The model under review builds one solid part; all positions refer to its coordinate system, in mm. Coordinates: 2 decimals unless noted, no trailing zeros. Put each result on its own line as item: value.
from build123d import *

# Parameters (mm, degrees)
SKETCH_1_R           = 2.1
SKETCH_1_R_2         = 3.15
EXTRUDE_1_DEPTH      = 5
SKETCH_2_OUTSIDE_W   = 463.828
SKETCH_2_OUTSIDE_H   = 463.828
SKETCH_2_OUTSIDE_W_2 = 280
SKETCH_2_OUTSIDE_H_2 = 360
CUT_EXTRUDE_2_DEPTH  = 10
SKETCH_3_R           = 2.1
CUT_EXTRUDE_3_DEPTH  = 229.089894559
CUT_EXTRUDE_5_DEPTH  = 10
FILLET_1_R           = 10


with BuildPart() as part:
    # 草图1 → 凸台-拉伸1 (new body)
    with BuildSketch(Plane(origin=(0, 0, 0), x_dir=(1, 0, 0), z_dir=(0, 1, 0))):
        Polygon((-180, -180), (180, -180), (180, -160), (141, -160), (141, -100), (180, -100), (180, -30), (141, -30), (141, 30), (180, 30), (180, 100), (141, 100), (141, 160), (180, 160), (180, 180), (-180, 180), (-180, 160), (-141, 160), (-141, 100), (-180, 100), (-180, 30), (-141, 30), (-141, -30), (-180, -30), (-180, -100), (-141, -100), (-141, -160), (-180, -160), align=None)
        with Locations(Location((-103, 145, 0), (0, 0, 270))):
            Circle(SKETCH_1_R, mode=Mode.SUBTRACT)
        with Locations(Location((-103, 115, 0), (0, 0, 90))):
            Circle(SKETCH_1_R, mode=Mode.SUBTRACT)
        with Locations(Location((-127, 145, 0), (0, 0, 90))):
            Circle(SKETCH_1_R, mode=Mode.SUBTRACT)
        with Locations(Location((-127, 115, 0), (0, 0, 270))):
            Circle(SKETCH_1_R, mode=Mode.SUBTRACT)
        with Locations(Location((103, 145, 0), (0, 0, 270))):
            Circle(SKETCH_1_R, mode=Mode.SUBTRACT)
        with Locations(Location((103, 115, 0), (0, 0, 90))):
            Circle(SKETCH_1_R, mode=Mode.SUBTRACT)
        with Locations(Location((127, 145, 0), (0, 0, 90))):
            Circle(SKETCH_1_R, mode=Mode.SUBTRACT)
        with Locations(Location((127, 115, 0), (0, 0, 270))):
            Circle(SKETCH_1_R, mode=Mode.SUBTRACT)
        with Locations(Location((127, -115, 0), (0, 0, 270))):
            Circle(SKETCH_1_R, mode=Mode.SUBTRACT)
        with Locations(Location((127, -145, 0), (0, 0, 90))):
            Circle(SKETCH_1_R, mode=Mode.SUBTRACT)
        with Locations(Location((103, -145, 0), (0, 0, 270))):
            Circle(SKETCH_1_R, mode=Mode.SUBTRACT)
        with Locations(Location((103, -115, 0), (0, 0, 90))):
            Circle(SKETCH_1_R, mode=Mode.SUBTRACT)
        with Locations(Location((-127, -115, 0), (0, 0, 270))):
            Circle(SKETCH_1_R, mode=Mode.SUBTRACT)
        with Locations(Location((-103, -115, 0), (0, 0, 90))):
            Circle(SKETCH_1_R, mode=Mode.SUBTRACT)
        with Locations(Location((-103, -145, 0), (0, 0, 270))):
            Circle(SKETCH_1_R, mode=Mode.SUBTRACT)
        with Locations(Location((-127, -145, 0), (0, 0, 90))):
            Circle(SKETCH_1_R, mode=Mode.SUBTRACT)
        with Locations(Location((17.5, -102, 0), (0, 0, 270))):
            Circle(SKETCH_1_R_2, mode=Mode.SUBTRACT)
        with Locations(Location((-17.5, -102, 0), (0, 0, 90))):
            Circle(SKETCH_1_R_2, mode=Mode.SUBTRACT)
        with Locations(Location((-17.5, -148, 0), (0, 0, 270))):
            Circle(SKETCH_1_R_2, mode=Mode.SUBTRACT)
        with Locations(Location((17.5, -148, 0), (0, 0, 90))):
            Circle(SKETCH_1_R_2, mode=Mode.SUBTRACT)
        with Locations(Location((-17.5, 148, 0), (0, 0, 270))):
            Circle(SKETCH_1_R_2, mode=Mode.SUBTRACT)
        with Locations(Location((17.5, 148, 0), (0, 0, 90))):
            Circle(SKETCH_1_R_2, mode=Mode.SUBTRACT)
        with Locations(Location((17.5, 102, 0), (0, 0, 270))):
            Circle(SKETCH_1_R_2, mode=Mode.SUBTRACT)
        with Locations(Location((-17.5, 102, 0), (0, 0, 90))):
            Circle(SKETCH_1_R_2, mode=Mode.SUBTRACT)
        with Locations(Location((-103, 15, 0), (0, 0, 270))):
            Circle(SKETCH_1_R, mode=Mode.SUBTRACT)
        with Locations(Location((-103, -15, 0), (0, 0, 90))):
            Circle(SKETCH_1_R, mode=Mode.SUBTRACT)
        with Locations(Location((-127, 15, 0), (0, 0, 90))):
            Circle(SKETCH_1_R, mode=Mode.SUBTRACT)
        with Locations(Location((-127, -15, 0), (0, 0, 270))):
            Circle(SKETCH_1_R, mode=Mode.SUBTRACT)
        with Locations(Location((127, 15, 0), (0, 0, 270))):
            Circle(SKETCH_1_R, mode=Mode.SUBTRACT)
        with Locations(Location((127, -15, 0), (0, 0, 90))):
            Circle(SKETCH_1_R, mode=Mode.SUBTRACT)
        with Locations(Location((103, 15, 0), (0, 0, 90))):
            Circle(SKETCH_1_R, mode=Mode.SUBTRACT)
        with Locations(Location((103, -15, 0), (0, 0, 270))):
            Circle(SKETCH_1_R, mode=Mode.SUBTRACT)
    extrude(amount=EXTRUDE_1_DEPTH)

    # 草图2 outside → 切除-拉伸2 (cut)
    with BuildSketch(Plane(origin=(0, 5, 0), x_dir=(1, 0, 0), z_dir=(0, 1, 0))):
        Rectangle(SKETCH_2_OUTSIDE_W, SKETCH_2_OUTSIDE_H)
        Rectangle(SKETCH_2_OUTSIDE_W_2, SKETCH_2_OUTSIDE_H_2, mode=Mode.SUBTRACT)
    extrude(amount=-CUT_EXTRUDE_2_DEPTH, mode=Mode.SUBTRACT)

    # 草图3 → 切除-拉伸3 (cut, through all)
    with BuildSketch(Plane(origin=(0, 5, 0), x_dir=(1, 0, 0), z_dir=(0, 1, 0))):
        with Locations(Location((-80, 80, 0), (0, 0, 270))):
            Circle(SKETCH_3_R)
        with Locations(Location((-120, 80, 0), (0, 0, 270))):
            Circle(SKETCH_3_R)
        with Locations(Location((-80, 120, 0), (0, 0, 270))):
            Circle(SKETCH_3_R)
        with Locations(Location((-80, -120, 0), (0, 0, 90))):
            Circle(SKETCH_3_R)
        with Locations(Location((-120, -80, 0), (0, 0, 90))):
            Circle(SKETCH_3_R)
        with Locations(Location((-80, -80, 0), (0, 0, 90))):
            Circle(SKETCH_3_R)
        with Locations(Location((80, -80, 0), (0, 0, 270))):
            Circle(SKETCH_3_R)
        with Locations(Location((120, -80, 0), (0, 0, 270))):
            Circle(SKETCH_3_R)
        with Locations(Location((80, -120, 0), (0, 0, 270))):
            Circle(SKETCH_3_R)
        with Locations(Location((80, 120, 0), (0, 0, 90))):
            Circle(SKETCH_3_R)
        with Locations(Location((120, 80, 0), (0, 0, 90))):
            Circle(SKETCH_3_R)
        with Locations(Location((80, 80, 0), (0, 0, 90))):
            Circle(SKETCH_3_R)
    extrude(amount=-CUT_EXTRUDE_3_DEPTH, mode=Mode.SUBTRACT)

    # 草图5 → 切除-拉伸5 (cut)
    with BuildSketch(Plane.XZ):
        with BuildLine():
            Line((-28, -45), (28, -45))
            ThreePointArc((28, -45), (29.414213562, -44.414213562), (30, -43))
            Line((30, -43), (30, -17))
            ThreePointArc((30, -17), (29.414213562, -15.585786438), (28, -15))
            Line((28, -15), (-28, -15))
            ThreePointArc((-28, -15), (-29.414213562, -15.585786438), (-30, -17))
            Line((-30, -17), (-30, -43))
            ThreePointArc((-30, -43), (-29.414213562, -44.414213562), (-28, -45))
        make_face()
    extrude(amount=-CUT_EXTRUDE_5_DEPTH, mode=Mode.SUBTRACT)

    # 圆角1
    fillet_1_edges = [part.edges().sort_by_distance(p)[0] for p in [
        (-140, 2.5, 180),
        (140, 2.5, 180),
        (-140, 2.5, -180),
        (140, 2.5, -180),
    ]]
    fillet(fillet_1_edges, radius=FILLET_1_R)


solid = part.part
Item 1: Consider section A-A on y = 3.8. Count the separate pieces of the cut face and the enclosed holes in it, and give its area (3 significant figures).
Answers below:
separate pieces: 1
enclosed holes: 45
area: 98,200 mm^2
Item 2: For line 1 (X direction, y = 2.7, z = -120); line 2 (X direction, y = 3.45, z = -115); line 3 (Z direction, x = 25.5, y = 3.85), list the stretches that pass through material, from the lowest coordinate up. Write a range as from..to.
Answers below:
line 1: -140..-82.1, -77.9..77.9, 82.1..140
line 2: -140..-129.1, -124.9..-105.1, -100.9..100.9, 105.1..124.9, 129.1..140
line 3: -180..-45, -15..180
Item 3: For pin 1 Ø3.5 at (x, z) = (-127, -15) entering from -Y, flat-tipped, find the tip position at first contact; note if it passes through.
Answers below:
pin 1: through
